Can you work these out from the model? Positions are in its coordinate system, mm. A direction names the side the tool comes from. Coordinates: 2 decimals unless noted, no trailing zeros. Order: outer loops, then holes, each group sorted by start corner. A loop starts at its lowest first (then second) coordinate and runs counter-clockwise, first axis right, second up. Notation, with made-up numbers: (-14.5, 3) -> (8.5, 3) arc R16 ccw to (8.5, 12) -> close; hole circle Ø1 at (70.25, 40). An arc over 180 degrees is marked (long way). Use a Markdown table: item, result. Add a question column.
1. Suppose I cut it at C-C, the plane x = 0.5. List the corners of the cut face in (y, z) for me, then the cut area to 3 significant figures.
2. For pin 1 Ø0.6 at (x, y) = (0, -1) entering from -Z; pin 2 Ø1.8 at (x, z) = (-1, -1) entering from -Y; pin 3 Ø4 at (x, y) = (0.5, 6.5) entering from +Z, each with a flat end and sliding along its axis, tell me the tip position at first contact or that it passes through.
3. For faces 1 (the flat face through (1, 6, 0)), 2 (the flat face through (0, 2, 1.75)), 3 (the flat face through (-0.4, 5.5, -0.82)), 4 (the flat face through (-0.4, 5.5, 0.82)), 5 (the flat face through (-1.8, 6, 0)), which set-ups out of +Z, -Z, +X, -X, +Y, -Y let a thin tool reach every point of the face, with its end or its side?
4. Suppose I cut it at D-D, the plane y = 6.5. List the corners of the cut face in (x, z) for me, then the cut area to 3 significant figures.
5. Suppose I cut it at B-B, the plane y = -1.75. List the corners of the cut face in (x, z) for me, then the cut area to 3 significant figures.
6. If I drill on line 1 along Y through (x, z) = (-3, 1.35); line 2 along Y through (x, z) = (-2.5, 0.1); line 3 along Z through (x, y) = (-1, 5.25), over which ranges is the centre line in solid material (lowest first)? Write a range as from..to.
7. Suppose I cut it at A-A, the plane z = 0.7. List the corners of the cut face in (x, y) for me.
```python
from build123d import *

# Parameters (mm, degrees)
SKETCH_1_W          = 8.5
SKETCH_1_H          = 3.5
EXTRUDE_1_DEPTH     = 4
SKETCH_2_W          = 3.6
SKETCH_2_H          = 1.64
EXTRUDE_2_DEPTH     = 4
SKETCH_3_W          = 1.8
SKETCH_3_H          = 1.64
CUT_EXTRUDE_1_DEPTH = 2
EXTRUDE_START       = -4
SKETCH_4_W          = 0.5
SKETCH_4_H          = 0.3
EXTRUDE_3_DEPTH     = 7.2


with BuildPart() as part:
    # 草图1 → 凸台-拉伸1 (new body)
    with BuildSketch(Plane(origin=(0, 0, 0), x_dir=(1, 0, 0), z_dir=(0, 1, 0))):
        Rectangle(SKETCH_1_W, SKETCH_1_H)
    extrude(amount=EXTRUDE_1_DEPTH)

    # 草图2 → 凸台-拉伸2 (add)
    with BuildSketch(Plane(origin=(0, 4, 0), x_dir=(1, 0, 0), z_dir=(0, 1, 0))):
        Rectangle(SKETCH_2_W, SKETCH_2_H)
    extrude(amount=EXTRUDE_2_DEPTH)

    # 草图3 → 切除-拉伸1 (cut)
    with BuildSketch(Plane(origin=(0, 8, 0), x_dir=(1, 0, 0), z_dir=(0, 1, 0))):
        with Locations((0.9, 0)):
            Rectangle(SKETCH_3_W, SKETCH_3_H)
    extrude(amount=-CUT_EXTRUDE_1_DEPTH, mode=Mode.SUBTRACT)

    # 草图4 → 凸台-拉伸3 (add)
    with BuildSketch(Plane.XZ.offset(EXTRUDE_START)):
        with Locations((2.5, 0)):
            Rectangle(SKETCH_4_W, SKETCH_4_H)
        Rectangle(SKETCH_4_W, SKETCH_4_H)
        with Locations((-2.5, 0)):
            Rectangle(SKETCH_4_W, SKETCH_4_H)
    extrude(amount=EXTRUDE_3_DEPTH)


solid = part.part
```
Worked out:
| question | item | result |
|---|---|---|
| 1 | outline | (0, -1.75) -> (4, -1.75) -> (4, -0.82) -> (6, -0.82) -> (6, 0.82) -> (4, 0.82) -> (4, 1.75) -> (0, 1.75) -> close |
| 1 | area | 17.3 mm² |
| 2 | pin 1 | stops at z = -0.15 |
| 2 | pin 2 | stops at y = 0 |
| 2 | pin 3 | stops at z = 0.82 |
| 3 | face 1 | +Z, -Z, +X, +Y |
| 3 | face 2 | +Z, +X, -X, +Y, -Y |
| 3 | face 3 | -Z, +X, -X, +Y |
| 3 | face 4 | +Z, +X, -X, +Y |
| 3 | face 5 | +Z, -Z, -X, +Y |
| 4 | outline | (-1.8, -0.82) -> (0, -0.82) -> (0, 0.82) -> (-1.8, 0.82) -> close |
| 4 | area | 2.95 mm² |
| 5 | outline | (-2.75, -0.15) -> (-2.25, -0.15) -> (-2.25, 0.15) -> (-2.75, 0.15) -> close; (-0.25, -0.15) -> (0.25, -0.15) -> (0.25, 0.15) -> (-0.25, 0.15) -> close; (2.25, -0.15) -> (2.75, -0.15) -> (2.75, 0.15) -> (2.25, 0.15) -> close |
| 5 | area | 0.450 mm² |
| 6 | line 1 | y = 0..4 |
| 6 | line 2 | y = -3.2..4 |
| 6 | line 3 | z = -0.82..0.82 |
| 7 | outline | (-4.25, 0) -> (4.25, 0) -> (4.25, 4) -> (1.8, 4) -> (1.8, 6) -> (0, 6) -> (0, 8) -> (-1.8, 8) -> (-1.8, 4) -> (-4.25, 4) -> close |
